Geometry check sheet. Reference: the model listing, model coordinates, mm. A direction names the side the tool comes from. Round coordinates to 2 decimals unless told otherwise and drop trailing zeros. Loops run counter-clockwise (first coordinate to the right, second up) from the corner with the lowest first, then second, coordinate; pieces in that order, holes last. Notation, with made-up numbers: (49, -33.75) -> (61, -33.75) arc R25 cw to (61, -1.75) -> close; hole circle Ø1 at (58, 78). An arc over 180 degrees is marked (long way). Use a Markdown table: item, result. Add a question column.
Q1. Material ranges on L1, parallel to X at y = -1.25, z = -2.25; L2, parallel to X at y = 7.5, z = 11.25; L3, parallel to Y at x = -9, z = -1.25, recorded low to high.
Q2. Gauge pin test, flat ends, axial feed: P1, Ø2, axis at x = -6, z = 0.5, coming from the +Y side; P2, Ø4, axis at y = 7, z = -10, coming from the -X side; P3, Ø12, axis at x = -22, y = 7.5, coming from the +Z side; P4, Ø10, axis at x = -10.5, z = 10, coming from the +Y side. Record the tip position at first contact, or that the pin passes through.
Q3. Sectioned sample at A-A, the plane y = 0. Enter the section's corners in (x, z), then the cut area to 3 significant figures.
Q4. Sectioned sample at C-C, the plane x = -3. Enter the section's corners in (y, z).
Q5. Set-up check for faces 1 (the face through (9, -2, 0)), 2 (the face through (17.5, 0, 0)), 3 (the face through (-38.86, -8.43, 4.38)): record each of +Z, -Z, +X, -X, +Y, -Y from which the full face is reachable in a straight line by a thin tool's end or side.
Q6. Sectioned sample at D-D, the plane y = 7.25. Enter the section's corners in (x, z), then the cut area to 3 significant figures.
```python
from build123d import *

# Parameters (mm, degrees)
F0_W   = 6
F0_H   = 9.5
F0_W_2 = 17.5
F0_H_2 = 2


with BuildPart() as f1:
    # F0 (on Front) → F1 (revolve)
    with BuildSketch(Plane.XZ):
        Polygon((0, 14.05), (-35.9, 14.05), (-35.9, 9.5), (-35.9, 0), (0, 0), (0, 2), align=None)
        with Locations((-38.9, 4.75)):
            Rectangle(F0_W, F0_H)
        with Locations((8.75, 1)):
            Rectangle(F0_W_2, F0_H_2)
    revolve(axis=Axis((-20.95, 0, 0), (-1, 0, 0)))


solid = f1.part
```
Values:
| question | item | result |
|---|---|---|
| 1 | L1 | -41.9 to 0 |
| 1 | L2 | -35.9 to 0 |
| 1 | L3 | -13.99 to 13.99 |
| 2 | P1 | y = 14.05 |
| 2 | P2 | x = -35.9 |
| 2 | P3 | z = 13.97 |
| 2 | P4 | y = 13.13 |
| 3 | outline | (-41.9, -9.5) -> (-35.9, -9.5) -> (-35.9, -14.05) -> (0, -14.05) -> (0, -2) -> (17.5, -2) -> (17.5, 2) -> (0, 2) -> (0, 14.05) -> (-35.9, 14.05) -> (-35.9, 9.5) -> (-41.9, 9.5) -> close |
| 3 | area | 1,190 mm^2 |
| 4 | outline | circle Ø28.1 at (0, 0) |
| 5 | face 1 | +X |
| 5 | face 2 | +Z, -Z, +X, +Y, -Y |
| 5 | face 3 | -X |
| 6 | outline | (-41.9, -6.14) -> (-35.9, -6.14) -> (-35.9, -12.03) -> (0, -12.03) -> (0, 12.03) -> (-35.9, 12.03) -> (-35.9, 6.14) -> (-41.9, 6.14) -> close |
| 6 | area | 938 mm^2 |
